```python
from build123d import *

# Parameters (mm, degrees)
F0_W     = 63.5
F0_H     = 63.5
F1_DEPTH = 25.4


with BuildPart() as f1:
    # F0 (on Front) → F1 (new body)
    with BuildSketch(Plane.XZ):
        with Locations((158.75, -209.55)):
            Rectangle(F0_W, F0_H)
        with BuildLine():
            Line((127, -177.8), (190.5, -177.8))
            Line((190.5, -177.8), (190.5, -127))
            Line((190.5, -127), (0, -127))
            ThreePointArc((0, -127), (-127, 0), (0, 127))
            Line((0, 127), (63.5, 127))
            Line((63.5, 127), (190.5, 127))
            Line((190.5, 127), (190.5, 177.8))
            Line((190.5, 177.8), (127, 177.8))
            Line((127, 177.8), (0, 177.8))
            Line((0, 177.8), (-24.553333, 177.8))
            ThreePointArc((-24.553333, 177.8), (-190.5, 0), (-24.553333, -177.8))
            Line((-24.553333, -177.8), (0, -177.8))
            Line((0, -177.8), (127, -177.8))
        make_face()
        with BuildLine():
            ThreePointArc((-24.553333, -177.8), (-12.276667, -178.223333), (0, -177.8))
            Line((0, -177.8), (-24.553333, -177.8))
        make_face()
        with BuildLine():
            ThreePointArc((0, 177.8), (-12.276667, 178.223333), (-24.553333, 177.8))
            Line((-24.553333, 177.8), (0, 177.8))
        make_face()
        with Locations((158.75, 209.55)):
            Rectangle(F0_W, F0_H)
    extrude(amount=F1_DEPTH)


solid = f1.part
```
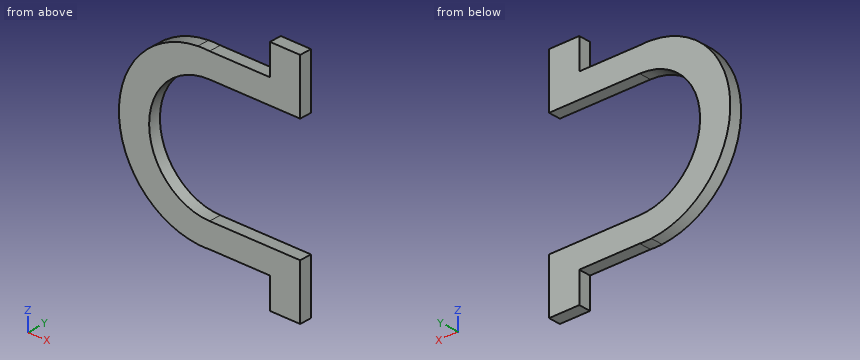
Geometry check sheet. Reference: the model listing, model coordinates, mm. Coordinates: 2 decimals unless noted, no trailing zeros. Loops run counter-clockwise (first coordinate to the right, second up) from the corner with the lowest first, then second, coordinate; pieces in that order, holes last.
Item 1: Sectioned sample at B-B, the plane y = -16.25. Record the boundary of the cut face in (x, z), then the cut area to 3 significant figures.
Item 2: Thickness scan on line 1 (X direction, y = -23.25, z = 207); line 2 (Z direction, x = 12.5, y = -17); line 3 (Z direction, x = -98, y = -17.5). Record the ranges inside material, lowest first.
Item 3: Sectioned sample at A-A, the plane x = 27.5. Record the boundary of the cut face in (y, z).
Item 4: Go/stop test with flat-tipped pins: pin 1 Ø12.5 at (x, y) = (99, -6.5) entering from +Z; pin 2 Ø12.5 at (x, y) = (64.5, -16.5) entering from -Z; pin 3 Ø7.5 at (y, z) = (-12.5, -220.5) entering from -X; pin 4 Ø3 at (x, z) = (134, 190.5) entering from +Y. Record where each tip stops, or that it passes through.
Item 5: Sectioned sample at D-D, the plane x = -63. Record the boundary of the cut face in (y, z).
Item 6: Sectioned sample at C-C, the plane z = 0. Record the boundary of the cut face in (x, y).
Check result:
1. outline: (-24.55, -177.8) arc R178.22 ccw to (0, -177.8) - (127, -177.8) - (127, -241.3) - (190.5, -241.3) - (190.5, -127) - (0, -127) arc R127 cw to (0, 127) - (190.5, 127) - (190.5, 241.3) - (127, 241.3) - (127, 177.8) - (0, 177.8) arc R178.22 ccw to (-24.55, 177.8) arc R178.22 ccw to start
1. area: 56,400 mm2
2. line 1: x = 127 to 190.5
2. line 2: z = -177.8 to -127, 127 to 177.8
2. line 3: z = -156.25 to -80.78, 80.78 to 156.25
3. outline: (-25.4, -177.8) - (0, -177.8) - (0, -127) - (-25.4, -127) - close; (-25.4, 127) - (0, 127) - (0, 177.8) - (-25.4, 177.8) - close
4. pin 1: stops at z = 177.8
4. pin 2: stops at z = -177.8
4. pin 3: stops at x = 127
4. pin 4: stops at y = 0
5. outline: (-25.4, -170.85) - (0, -170.85) - (0, -110.27) - (-25.4, -110.27) - close; (-25.4, 110.27) - (0, 110.27) - (0, 170.85) - (-25.4, 170.85) - close
6. outline: (-190.5, -25.4) - (-127, -25.4) - (-127, 0) - (-190.5, 0) - close
